from build123d import *

# Parameters (mm, degrees)
F0_R     = 7.4
F1_DEPTH = 10
F2_W     = 14.8
F2_H     = 14.8
F3_DEPTH = 25
F5_DEPTH = 12.5


with BuildPart() as f1:
    # F0 (on Top) → F1 (new body)
    with BuildSketch(Plane.XY):
        Circle(F0_R)
    extrude(amount=-F1_DEPTH)

    # F2 (on face) → F3 (join)
    with BuildSketch(Plane.XY):
        Rectangle(F2_W, F2_H)
    extrude(amount=F3_DEPTH)

    # F4 (on Front) → F5 (cut, symmetric)
    with BuildSketch(Plane.XZ):
        with BuildLine():
            ThreePointArc((-1, 17.0277164746), (-2.5566090824, 9.7310169777), (4.15, 13))
            ThreePointArc((4.15, 13), (3.2689830223, 15.5566090824), (1, 17.0277164746))
            Line((1, 17.0277164746), (1, 13))
            Line((1, 13), (-1, 13))
            Line((-1, 13), (-1, 17.0277164746))
        make_face()
        with BuildLine():
            Line((1, 13), (1, 17.0277164746))
            ThreePointArc((1, 17.0277164746), (0, 17.15), (-1, 17.0277164746))
            Line((-1, 17.0277164746), (-1, 13))
            Line((-1, 13), (1, 13))
        make_face()
        with BuildLine():
            ThreePointArc((-1, 17.0277164746), (0, 17.15), (1, 17.0277164746))
            Line((1, 17.0277164746), (1, 25))
            Line((1, 25), (-1, 25))
            Line((-1, 25), (-1, 17.0277164746))
        make_face()
    extrude(amount=F5_DEPTH, both=True, mode=Mode.SUBTRACT)


solid = f1.part
Verification items for the finished model (mm, model axes). A direction names the side the tool comes from. Coordinates: 2 decimals unless noted, no trailing zeros. Write each loop counter-clockwise with the first axis right and the second up, starting at its lowest first coordinate (ties: lowest second). Pieces come first, ordered by that corner, then holes. Notation, with made-up numbers: M 31,57.5 L 60,57.5 A29 cw 60,85.5 Z; hole C -23.5,22.25 d9. An arc over 180 degrees is marked long. One line per question, with ' | ' between items.
1) Sectioned sample at D-D on x = -3.5. Record the cut outline in (y, z), then the cut area to 3 significant figures.
Solutions:
outline: M -7.4,0 L -6.52,0 L -6.52,-10 L 6.52,-10 L 6.52,0 L 7.4,0 L 7.4,10.77 L -7.4,10.77 Z; M -7.4,15.23 L 7.4,15.23 L 7.4,25 L -7.4,25 Z | area: 434 mm^2
2) Access from +Z, -Z, +X, -X, +Y, -Y to the whole of each face (thin tool, end or side, straight path). Record for faces 1 (the face through (-1.604, -7.224, -4.93)), 2 (the face through (-1, 0, 21)), 3 (the face through (-6, 6, 0)), 4 (the face through (6, -6, 0)), 5 (the face through (6, 6, 0)).
Solutions:
face 1: -Z | face 2: +Z, +Y, -Y | face 3: -Z, -X, +Y | face 4: -Z, +X, -Y | face 5: -Z, +X, +Y
3) Material ranges on L1, parallel to X at y = 2, z = 13; L2, parallel to Z at x = 6, y = 6; L3, parallel to X at y = -5, z = 17.5, recorded low to high.
Solutions:
L1: -7.4 to -4.15, 4.15 to 7.4 | L2: 0 to 25 | L3: -7.4 to -1, 1 to 7.4
4) Sectioned sample at C-C on y = 2.25. Record the cut outline in (x, z), then the cut area to 3 significant figures.
Solutions:
outline: M -7.4,0 L -7.05,0 L -7.05,-10 L 7.05,-10 L 7.05,0 L 7.4,0 L 7.4,25 L 1,25 L 1,17.03 A4.15 cw long -1,17.03 L -1,25 L -7.4,25 Z | area: 441 mm^2
5) Depth check by flat-ended pin: pin 1 Ø8 at (x, z) = (-5, -5) entering from +Y. Enter the tip coordinate at first touch or a pass-through.
Solutions:
pin 1: y = 7.33
6) Sectioned sample at A-A on z = 22. Record the cut outline in (x, y), then the cut area to 3 significant figures.
Solutions:
outline: M -7.4,-7.4 L -1,-7.4 L -1,7.4 L -7.4,7.4 Z; M 1,-7.4 L 7.4,-7.4 L 7.4,7.4 L 1,7.4 Z | area: 189 mm^2
7) Sectioned sample at B-B on x = 2.5. Record the cut outline in (y, z), then the cut area to 3 significant figures.
Solutions:
outline: M -7.4,0 L -6.96,0 L -6.96,-10 L 6.96,-10 L 6.96,0 L 7.4,0 L 7.4,9.69 L -7.4,9.69 Z; M -7.4,16.31 L 7.4,16.31 L 7.4,25 L -7.4,25 Z | area: 411 mm^2
